Geometry check sheet. Reference: drawing and pictorial views, mm from the part's lowest x, y, z. Round coordinates to 2 decimals unless told otherwise and drop trailing zeros. Order: outer loops, then holes, each group sorted by start corner. A loop starts at its lowest first (then second) coordinate and runs counter-clockwise, first axis right, second up.
Q1. Cross-section at D-D on y = 5.25. Record the cut outline in (x, z).
Q2. Depth check by flat-ended pin: P1, Ø2, axis at y = 6.5, z = 6.5, coming from the +X side. Enter the tip coordinate at first touch or a pass-through.
Q3. Scan lines: probe 1 along Y at (x, z) = (14.25, 1.5); probe 2 along X at (y, z) = (3.5, 3.25); probe 3 along X at (y, z) = (3, 0.75) (3 decimals). Record each from-to range of solid material in increasing order.
Q4. Cross-section at B-B on x = 2.25. Record the cut outline in (y, z).
Q5. Cross-section at C-C on z = 2. Record the cut outline in (x, y) (3 decimals).
Q6. Cross-section at A-A on y = 4.05. Record the cut outline in (x, z) (3 decimals).
Q7. Mould release check, pull along X, two halves, no side actions. Record for the marked faces 1, 2, 3 and 4: +X half, -X half, draft (parallel to the pull), parting line (faces both ways), or undercut.
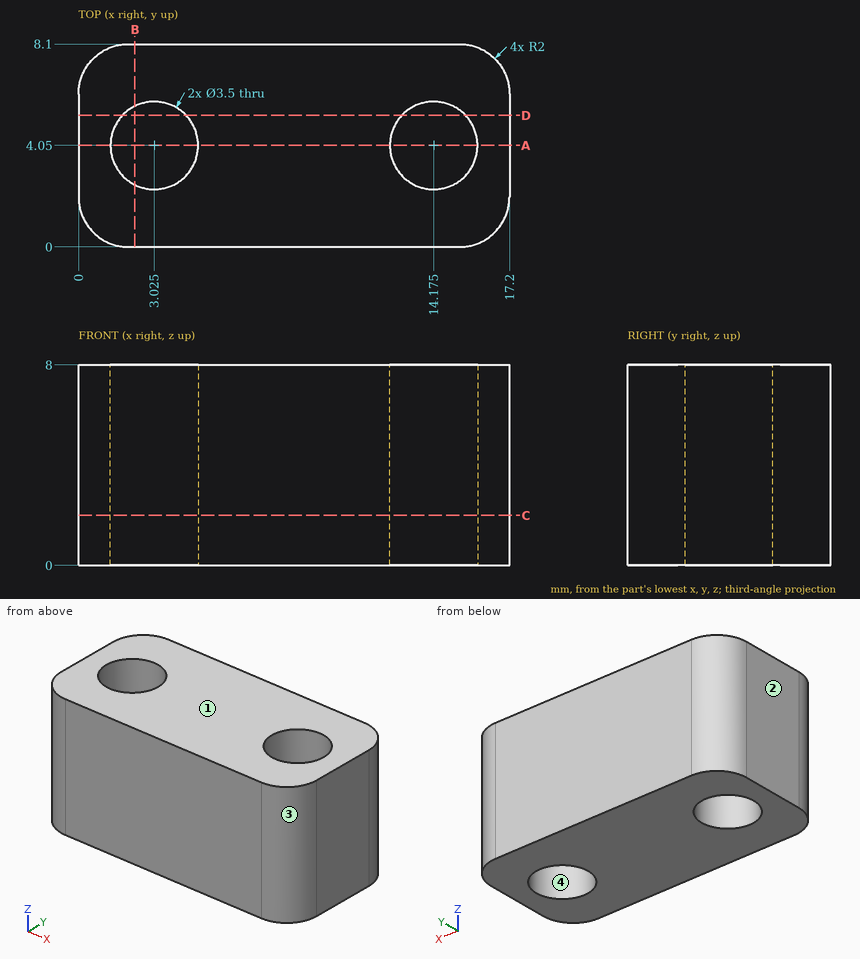
Results found:
1. outline: (0, 0) - (1.75, 0) - (1.75, 8) - (0, 8) - close; (4.3, 0) - (12.9, 0) - (12.9, 8) - (4.3, 8) - close; (15.45, 0) - (17.2, 0) - (17.2, 8) - (15.45, 8) - close
2. P1: stops at x = 17.2
3. probe 1: y = 0 to 2.3, 5.8 to 8.1
3. probe 2: x = 0 to 1.36, 4.69 to 12.51, 15.84 to 17.2
3. probe 3: x = 0 to 1.625, 4.425 to 12.775, 15.575 to 17.2
4. outline: (0, 0) - (2.48, 0) - (2.48, 8) - (0, 8) - close; (5.62, 0) - (8.1, 0) - (8.1, 8) - (5.62, 8) - close
5. outline: (0, 2) arc R2 ccw to (2, 0) - (15.2, 0) arc R2 ccw to (17.2, 2) - (17.2, 6.1) arc R2 ccw to (15.2, 8.1) - (2, 8.1) arc R2 ccw to (0, 6.1) - close; hole circle Ø3.5 at (3.025, 4.05); hole circle Ø3.5 at (14.175, 4.05)
6. outline: (0, 0) - (1.275, 0) - (1.275, 8) - (0, 8) - close; (4.775, 0) - (12.425, 0) - (12.425, 8) - (4.775, 8) - close; (15.925, 0) - (17.2, 0) - (17.2, 8) - (15.925, 8) - close
7. face 1: draft
7. face 2: -X half
7. face 3: +X half
7. face 4: undercut
